For this review, use the dimensioned drawing (mm, ordinates from the lowest corner) and the shaded views. A direction names the side the tool comes from. Round coordinates to 2 decimals unless told otherwise and drop trailing zeros. Loops run counter-clockwise (first coordinate to the right, second up) from the corner with the lowest first, then second, coordinate; pieces in that order, holes last.
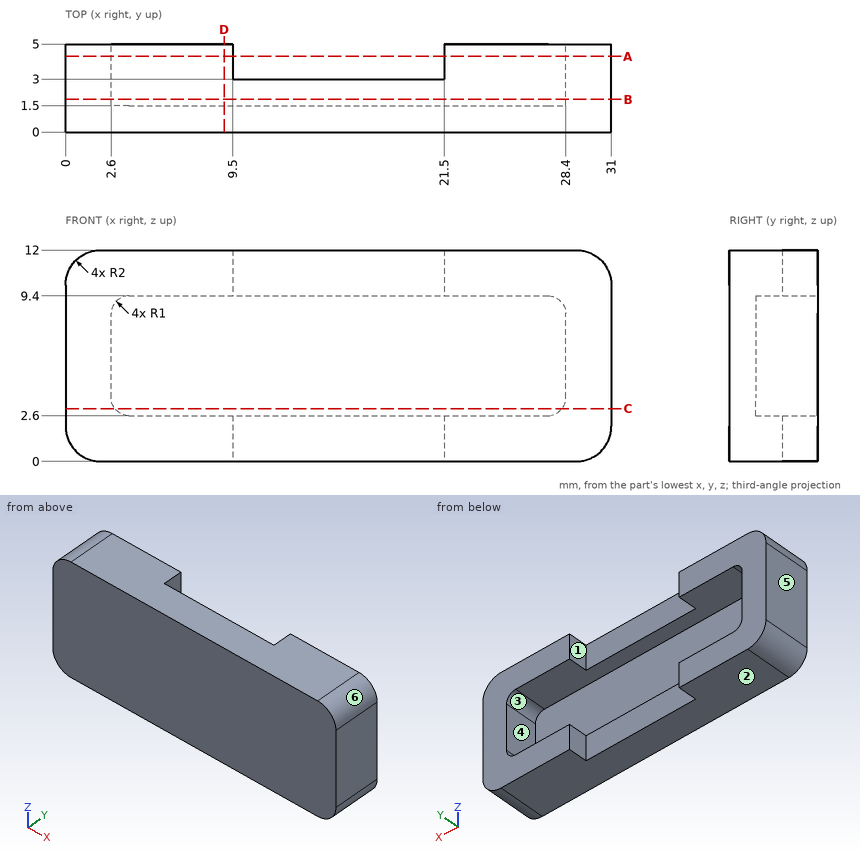
(1) For L1, parallel to X at y = 2.25, z = 4; L2, parallel to Z at x = 6, y = 4.55; L3, parallel to Y at x = 19.5, z = 9, list the stretches that pass through material, from the lowest coordinate up.
(2) For the marked faces 1, 2 and 3, list the 3-axis set-ups (+Z, -Z, +X, -X, +Y, -Y) from which the entire face can be reached by the end or side of a thin tool; tool diameter is ignored.
(3) Add section C-C (z = 3). Give the boundary of the cut face in (x, y).
(4) The part is to be moulded in two halves that separate along Z. For the marked faces 4, 5 and 6, say which applies: pulls with the +Z half, pulls with the -Z half, needs draft (parallel to the pull), parting line crosses it, or undercut.
(5) Insertion check: pin 1 Ø1.3 at (x, z) = (13.5, 1.5) entering from +Y; pin 2 Ø5.5 at (x, z) = (18.5, 6) entering from +Y; pin 3 Ø0.6 at (y, z) = (3.5, 10.5) entering from -X. Each pin has a flat end and moves straight along its axis. Give the tip position at first contact, or say it passes through.
(6) Add section D-D (x = 9). Give the boundary of the cut face in (y, z), plus the area to 3 significant figures.
(7) Add section A-A (y = 4.3). Give the boundary of the cut face in (x, z), plus the area to 3 significant figures.
(8) Add section B-B (y = 1.85). Give the boundary of the cut face in (x, z).
Outcome:
1. L1: x = 0 to 2.6, 28.4 to 31
1. L2: z = 0 to 2.6, 9.4 to 12
1. L3: y = 0 to 1.5
2. face 1: +Z, -Z, +Y
2. face 2: -Z, +X, -X, +Y, -Y
2. face 3: +Y
3. outline: (0, 0) - (31, 0) - (31, 5) - (28.2, 5) - (28.2, 1.5) - (2.8, 1.5) - (2.8, 5) - (0, 5) - close
4. face 4: undercut
4. face 5: needs draft
4. face 6: pulls with the +Z half
5. pin 1: stops at y = 3
5. pin 2: stops at y = 1.5
5. pin 3: stops at x = 0.01
6. outline: (0, 0) - (5, 0) - (5, 2.6) - (1.5, 2.6) - (1.5, 9.4) - (5, 9.4) - (5, 12) - (0, 12) - close
6. area: 36.2 mm2
7. outline: (0, 2) arc R2 ccw to (2, 0) - (9.5, 0) - (9.5, 2.6) - (3.6, 2.6) arc R1 cw to (2.6, 3.6) - (2.6, 8.4) arc R1 cw to (3.6, 9.4) - (9.5, 9.4) - (9.5, 12) - (2, 12) arc R2 ccw to (0, 10) - close; (21.5, 0) - (29, 0) arc R2 ccw to (31, 2) - (31, 10) arc R2 ccw to (29, 12) - (21.5, 12) - (21.5, 9.4) - (27.4, 9.4) arc R1 cw to (28.4, 8.4) - (28.4, 3.6) arc R1 cw to (27.4, 2.6) - (21.5, 2.6) - close
7. area: 132 mm2
8. outline: (0, 2) arc R2 ccw to (2, 0) - (29, 0) arc R2 ccw to (31, 2) - (31, 10) arc R2 ccw to (29, 12) - (2, 12) arc R2 ccw to (0, 10) - close; hole (2.6, 3.6) arc R1 ccw to (3.6, 2.6) - (27.4, 2.6) arc R1 ccw to (28.4, 3.6) - (28.4, 8.4) arc R1 ccw to (27.4, 9.4) - (3.6, 9.4) arc R1 ccw to (2.6, 8.4) - close
